The listing builds one solid part. Answer for the finished solid, in the listing's coordinates (mm). Coordinates: 2 decimals unless noted, no trailing zeros. Loops run counter-clockwise (first coordinate to the right, second up) from the corner with the lowest first, then second, coordinate; pieces in that order, holes last. Notation, with made-up numbers: M 7,12.5 L 51,12.5 A11 cw 51,30.5 Z; hole C -2.75,67.25 d3. An arc over 180 degrees is marked long. Answer in a Markdown table with one row per item. Add a question column.
from build123d import *

# Parameters (mm, degrees)
ESQUISSE1_W        = 172.93
ESQUISSE1_H        = 273
ESQUISSE1_R        = 1.5
ESQUISSE1_W_2      = 87
ESQUISSE1_H_2      = 152
ESQUISSE1_W_3      = 52
ESQUISSE1_H_3      = 28
BOSS_EXTRU_1_DEPTH = 4
CONG_1_R           = 3
D_GAGEMENT_M31_D   = 3.4


with BuildPart() as part:
    # Esquisse1 → Boss.-Extru.1 (new body)
    with BuildSketch(Plane.XY):
        with Locations((86.465, 136.5)):
            Rectangle(ESQUISSE1_W, ESQUISSE1_H)
        with Locations((7.93, 236.5)):
            Circle(ESQUISSE1_R, mode=Mode.SUBTRACT)
        with Locations((7.93, 70.5)):
            Circle(ESQUISSE1_R, mode=Mode.SUBTRACT)
        with Locations((157.93, 236.5)):
            Circle(ESQUISSE1_R, mode=Mode.SUBTRACT)
        with Locations((86.5, 151)):
            Rectangle(ESQUISSE1_W_2, ESQUISSE1_H_2, mode=Mode.SUBTRACT)
        with Locations((72.93, 46)):
            Rectangle(ESQUISSE1_W_3, ESQUISSE1_H_3, mode=Mode.SUBTRACT)
    extrude(amount=BOSS_EXTRU_1_DEPTH)

    # Congé1
    cong_1_edges = [part.edges().sort_by_distance(p)[0] for p in [
        (43, 227, 2),
        (43, 75, 2),
        (130, 75, 2),
        (130, 227, 2),
        (46.93, 60, 2),
        (46.93, 32, 2),
        (98.93, 32, 2),
        (98.93, 60, 2),
        (0, 273, 2),
        (172.93, 273, 2),
        (172.93, 0, 2),
        (0, 0, 2),
    ]]
    fillet(cong_1_edges, radius=CONG_1_R)

    # Dégagement M31 (through all)
    with Locations(Plane.XY.offset(4)):
        with Locations((7.93, 236.5), (7.93, 70.5), (157.93, 236.5)):
            Hole(D_GAGEMENT_M31_D / 2)


solid = part.part
(1) A cutting plane is placed at C-C (z = 0.7). Give the vertices of the cut face in (x, y), plus the area to 3 significant figures.
(2) A cutting plane is placed at B-B (x = 107). Give the vertices of the cut face in (y, z).
(3) A cutting plane is placed at D-D (x = 56.5). Give the vertices of the cut face in (y, z).
(4) Straight lines are drawn through the part: line 1 (X direction, y = 236.5, z = 1.05); line 2 (Y direction, x = 7.93, z = 2.9); line 3 (Y direction, x = 76, z = 2.8). For each, find the intervals that lie inside material, in ascending order.
(5) A cutting plane is placed at A-A (y = 38). Give the vertices of the cut face in (x, z), plus the area to 3 significant figures.
Solved:
| question | item | result |
|---|---|---|
| 1 | outline | M 0,3 A3 ccw 3,0 L 169.93,0 A3 ccw 172.93,3 L 172.93,270 A3 ccw 169.93,273 L 3,273 A3 ccw 0,270 Z; hole C 7.93,70.5 d3.4; hole C 7.93,236.5 d3.4; hole M 43,78 A3 ccw 46,75 L 127,75 A3 ccw 130,78 L 130,224 A3 ccw 127,227 L 46,227 A3 ccw 43,224 Z; hole M 46.93,35 A3 ccw 49.93,32 L 95.93,32 A3 ccw 98.93,35 L 98.93,57 A3 ccw 95.93,60 L 49.93,60 A3 ccw 46.93,57 Z; hole C 157.93,236.5 d3.4 |
| 1 | area | 32,500 mm² |
| 2 | outline | M 0,0 L 75,0 L 75,4 L 0,4 Z; M 227,0 L 273,0 L 273,4 L 227,4 Z |
| 3 | outline | M 0,0 L 32,0 L 32,4 L 0,4 Z; M 60,0 L 75,0 L 75,4 L 60,4 Z; M 227,0 L 273,0 L 273,4 L 227,4 Z |
| 4 | line 1 | x = 0 to 6.23, 9.63 to 156.23, 159.63 to 172.93 |
| 4 | line 2 | y = 0 to 68.8, 72.2 to 234.8, 238.2 to 273 |
| 4 | line 3 | y = 0 to 32, 60 to 75, 227 to 273 |
| 5 | outline | M 0,0 L 46.93,0 L 46.93,4 L 0,4 Z; M 98.93,0 L 172.93,0 L 172.93,4 L 98.93,4 Z |
| 5 | area | 484 mm² |
